CAD build for the part. Positions are in the model's coordinates, mm. Face numbers are marked on the shaded views. A direction names the side the tool comes from. Round coordinates to 2 decimals unless told otherwise and drop trailing zeros. Loops run counter-clockwise (first coordinate to the right, second up) from the corner with the lowest first, then second, coordinate; pieces in that order, holes last. Notation, with made-up numbers: (88.5, 75) -> (132.5, 75) arc R18 ccw to (132.5, 96) -> close; hole circle Ø8 at (20.5, 73). An arc over 180 degrees is marked (long way). Answer as CSV lines item,"result".
Solid Edge part; units mm, degrees
sketch "Sketch1" plane through (0, 0, 0) normal (0, 0, 1) x (1, 0, 0)
  line L0 (0, 19.5) -> (0, 6.5)
  line L1 (13, 6.5) -> (13, 19.5)
  arc A0 (13, 6.5) -> (0, 6.5) centre (6.5, 6.5) cw
  arc A1 (0, 19.5) -> (13, 19.5) centre (6.5, 19.5) cw
extrude "Protrusion1" add sketch "Sketch1" along normal blind 6.5
sketch "Sketch2" plane through (6.5, 0, 0) normal (1, 0, 0) x (0, 1, 0)
  line L0 (3.5, 5.5) -> (3.5, 6.5)
  line L1 (3.5, 6.5) -> (6.5, 6.5)
  line L2 (6.5, 1) -> (6.5, 6.5)
  line L3 (3.5, 1) -> (6.5, 1)
  line L4 (3.5, 1) -> (2.6811, 3.25)
  line L5 (3.5, 5.5) -> (2.6811, 3.25)
revolve "RevolvedCutout1" cut sketch "Sketch2" angle 360 about axis through (6.5, 6.5, 1) along (0, 0, 1)
chamfer "Chaflán_38" distance 0.75 angle 45 1 edges at (6.5, 3.5, 6.5)
pattern_linear "Pattern1" count 2 spacing 13 along (0, 1, 0) of "RevolvedCutout1", "Chaflán_38"
chamfer "Chaflán_39" distance 1.5 angle 45 8 edges at (13, 13, 6.5) (6.5, 0, 6.5) (0, 13, 6.5) (6.5, 26, 6.5) (13, 13, 0) (6.5, 0, 0) (0, 13, 0) (6.5, 26, 0)
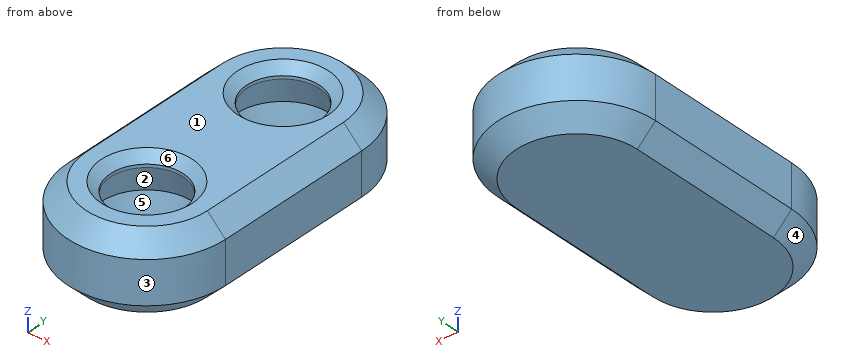
Q1. Slice it at A-A, the plane x = 6.5. Give the cut face in (y, z), and give its area (3 significant figures).
Results:
outline,"(0, 1.5) -> (1.5, 0) -> (24.5, 0) -> (26, 1.5) -> (26, 5) -> (24.5, 6.5) -> (23.25, 6.5) -> (22.5, 5.75) -> (22.5, 5.5) -> (23.32, 3.25) -> (22.5, 1) -> (16.5, 1) -> (15.68, 3.25) -> (16.5, 5.5) -> (16.5, 5.75) -> (15.75, 6.5) -> (10.25, 6.5) -> (9.5, 5.75) -> (9.5, 5.5) -> (10.32, 3.25) -> (9.5, 1) -> (3.5, 1) -> (2.68, 3.25) -> (3.5, 5.5) -> (3.5, 5.75) -> (2.75, 6.5) -> (1.5, 6.5) -> (0, 5) -> close"
area,"90.0 mm2"
Q2. Slice it at C-C, the plane z = 4.25. Give the cut face in (x, y).
Results:
outline,"(0, 6.5) arc R6.5 ccw to (13, 6.5) -> (13, 19.5) arc R6.5 ccw to (0, 19.5) -> close; hole circle Ø6.91 at (6.5, 6.5); hole circle Ø6.91 at (6.5, 19.5)"
Q3. Tool access for the marked faces 5 and 6: list every direction of +Z, -Z, +X, -X, +Y, -Y with a clear straight run to the whole face (end or side of a thin tool).
Results:
face 5,"none"
face 6,"+Z"
Q4. Probe L1, parallel to Y at x = 8, z = 5.5; L2, parallel to Z at x = 6, y = 3.75; L3, parallel to X at y = 19.5, z = 5.7. List the from-to ranges inside material, lowest first. Write a range as [from, to].
Results:
L1,"[0.69, 3.9], [9.1, 16.9], [22.1, 25.31]"
L2,"[0, 1]"
L3,"[0.7, 3.5], [9.5, 12.3]"
Q5. Drop flat-ended pins along their axis: pin 1 Ø5 at (x, y) = (6.5, 19.5) entering from +Z; pin 2 Ø2 at (y, z) = (22.5, 4.5) entering from +X; pin 3 Ø1.5 at (x, z) = (2, 4.5) entering from +Y. Give the stop position or say it passes through.
Results:
pin 1,"z = 1"
pin 2,"x = 12.68"
pin 3,"y = 24.81"
Q6. Two-plate mould, pull along Z, no slides. Class the marked faces 1, 2, 3 and 4: pulls with the +Z half, pulls with the -Z half, needs draft (parallel to the pull), parting line crosses it, or undercut.
Results:
face 1,"pulls with the +Z half"
face 2,"undercut"
face 3,"needs draft"
face 4,"pulls with the -Z half"
Q7. Slice it at B-B, the plane y = 13.5. Give the cut face in (x, z).
Results:
outline,"(0, 1.5) -> (1.5, 0) -> (11.5, 0) -> (13, 1.5) -> (13, 5) -> (11.5, 6.5) -> (1.5, 6.5) -> (0, 5) -> close"
